from build123d import *

# Parameters (mm, degrees)
F2_R     = 4
F3_DEPTH = 15.001
F4_R     = 5
F5_DEPTH = 15.001


with BuildPart() as f1:
    # F0 (on Front) → F1 (revolve)
    with BuildSketch(Plane.XZ):
        Polygon((0, -7.5), (0, 7.5), (-25, 7.5), (-25, 5), (-20, 5), (-20, -5), (-25, -5), (-25, -7.5), align=None)
    revolve(axis=Axis((0, 0, 0), (0, 0, -1)))

    # F2 (on face) → F3 (cut, through all)
    with BuildSketch(Plane.XY.offset(7.5)):
        Circle(F2_R)
    extrude(amount=-F3_DEPTH, mode=Mode.SUBTRACT)

    # F4 (on face) → F5 (cut, through all)
    with BuildSketch(Plane.XY.offset(7.5)):
        with Locations((-12, 0)):
            Circle(F4_R)
        with Locations((0, 12)):
            Circle(F4_R)
        with Locations((12, 0)):
            Circle(F4_R)
        with Locations((0, -12)):
            Circle(F4_R)
    extrude(amount=-F5_DEPTH, mode=Mode.SUBTRACT)


solid = f1.part
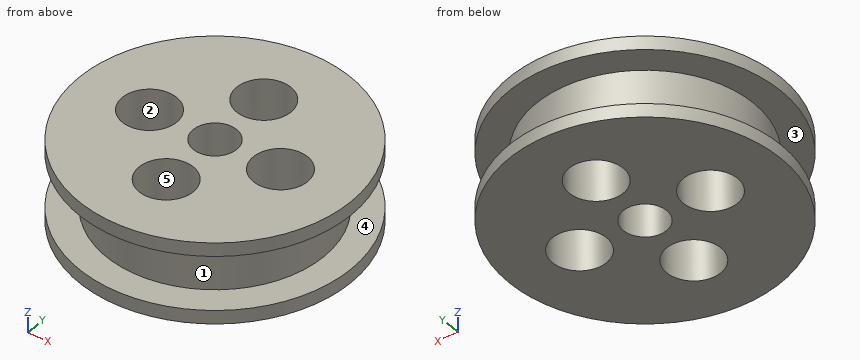
Can you work these out from the model? Positions are in its coordinate system, mm. Face numbers are marked on the shaded views. A direction names the side the tool comes from. Give positions to 0.01 mm unless a question says otherwise; leave off trailing zeros. Order: outer loops, then holes, each group sorted by start corner. A loop starts at its lowest first (then second) coordinate and runs counter-clockwise, first axis right, second up. Notation, with made-up numbers: M -11,18.25 L 38,18.25 A17 ccw 38,26.25 Z; hole C 71.5,-25.75 d7. An arc over 180 degrees is marked long. One line per question, with ' | ' between items.
Item 1: Suppose I cut it at C-C, the plane x = -12. Write out the boundary of the cut face in (y, z).
Answer block:
outline: M -21.93,-7.5 L -5,-7.5 L -5,7.5 L -21.93,7.5 L -21.93,5 L -16,5 L -16,-5 L -21.93,-5 Z; M 5,-7.5 L 21.93,-7.5 L 21.93,-5 L 16,-5 L 16,5 L 21.93,5 L 21.93,7.5 L 5,7.5 Z
Item 2: Suppose I cut it at B-B, the plane z = 6.25. Write out the boundary of the cut face in (x, y), then the cut area to 3 significant figures.
Answer block:
outline: C 0,0 d50; hole C -12,0 d10; hole C 0,-12 d10; hole C 0,12 d10; hole C 0,0 d8; hole C 12,0 d10 | area: 1,600 mm2
Item 3: For the marked faces 4 and 5, which set-ups out of +Z, -Z, +X, -X, +Y, -Y let a thin tool reach every point of the face, with its end or its side?
Answer block:
face 4: none | face 5: +Z, -Z
Item 4: Please list where these lines run through material, in increasing order: L1, parallel to Y at x = 0, z = -1.75; L2, parallel to Y at x = -2, z = 6.5; L3, parallel to X at y = 3, z = 5.25.
Answer block:
L1: y = -20 to -17, -7 to -4, 4 to 7, 17 to 20 | L2: y = -24.92 to -16.58, -7.42 to -3.46, 3.46 to 7.42, 16.58 to 24.92 | L3: x = -24.82 to -16, -8 to -2.65, 2.65 to 8, 16 to 24.82
Item 5: I'm going to push flat-ended pins straight in: pin 1 Ø1.5 at (y, z) = (17.5, 0.5) entering from -X; pin 2 Ø4 at (y, z) = (-7.5, 4) entering from -X; pin 3 Ø4 at (y, z) = (-19.5, 1) entering from +X. Where does each tip first touch, or does it pass through?
Answer block:
pin 1: stops at x = -10.93 | pin 2: stops at x = -24.33 | pin 3: stops at x = 9.68
Item 6: Suppose I cut it at A-A, the plane y = 0. Write out the boundary of the cut face in (x, z), then the cut area to 3 significant figures.
Answer block:
outline: M -25,-7.5 L -17,-7.5 L -17,7.5 L -25,7.5 L -25,5 L -20,5 L -20,-5 L -25,-5 Z; M -7,-7.5 L -4,-7.5 L -4,7.5 L -7,7.5 Z; M 4,-7.5 L 7,-7.5 L 7,7.5 L 4,7.5 Z; M 17,-7.5 L 25,-7.5 L 25,-5 L 20,-5 L 20,5 L 25,5 L 25,7.5 L 17,7.5 Z | area: 230 mm2
Item 7: We'd pull the mould along X, two halves only. Please class the marked faces 1, 2 and 3: released by +X, released by -X, zero draft, split by the parting line, or undercut.
Answer block:
face 1: split by the parting line | face 2: undercut | face 3: zero draft
